Work out the finished part from the listing and answer in its coordinate system (mm). A direction names the side the tool comes from. Coordinates: 2 decimals unless noted, no trailing zeros. Order: outer loops, then holes, each group sorted by start corner. A loop starts at its lowest first (then second) coordinate and runs counter-clockwise, first axis right, second up. Notation, with made-up numbers: M 40.5,-20.75 L 62.5,-20.75 A8 cw 62.5,-14.75 Z; hole C -34.75,5.5 d2. An arc over 180 degrees is marked long. Use a Markdown table: item, result.
from build123d import *

# Parameters (mm, degrees)
F3_DEPTH = 0.5
F4_DEPTH = 0.5
F2_R     = 11.884128
F5_DEPTH = 0.5
F6_R     = 4.759852
F7_DEPTH = 1


with BuildPart() as f3:
    # F0 (on Front) → F3 (new body, symmetric)
    with BuildSketch(Plane.XZ):
        Polygon((0.76961, 25.458554), (-0.685163, 25.458554), (-11.722775, 0), (11.791914, 0), align=None)
    extrude(amount=F3_DEPTH, both=True)

    # F1 (on Right) → F4 (join, symmetric)
    with BuildSketch(Plane.YZ):
        Polygon((0, 25.482798), (-0.616243, 25.482798), (-10.725138, 0), (0, 0), (11.086991, 0), (0.637034, 25.482798), align=None)
    extrude(amount=F4_DEPTH, both=True)

    # F2 (on Top) → F5 (join)
    with BuildSketch(Plane.XY):
        Circle(F2_R)
    extrude(amount=-F5_DEPTH)

    # F6 (on face) → F7 (join)
    with BuildSketch(Plane.XY.offset(25.482798)):
        Circle(F6_R)
    extrude(amount=F7_DEPTH)


solid = f3.part
(1) A cutting plane is placed at D-D (x = 0). Determine the outline of the cut face in (y, z), then the cut area to 3 significant figures.
Conclusion:
| item | result |
|---|---|
| outline | M -11.88,-0.5 L 11.88,-0.5 L 11.88,0 L 11.09,0 L 0.64,25.48 L 4.76,25.48 L 4.76,26.48 L -4.76,26.48 L -4.76,25.48 L -0.62,25.48 L -10.73,0 L -11.88,0 Z |
| area | 315 mm2 |
(2) Straight lines are drawn through the part: L1, parallel to Z at x = -1, y = -2.25; L2, parallel to X at y = -5, z = 14; L3, parallel to Z at x = -2.5, y = 4.5. For each, find the intervals that lie inside material, in ascending order.
Conclusion:
| item | result |
|---|---|
| L1 | -0.5 to 0, 25.48 to 26.48 |
| L2 | -0.5 to 0.5 |
| L3 | -0.5 to 0 |
(3) Determine the mould class of faces 1 (the flat face through (0, 0, 26.483)), 2 (the flat face through (0.007, 5.935, 12.563)), 3 (the flat face through (0, 0, -0.5)), 4 (the cylindrical face through (4.54, 1.43, 25.98)) for opening direction Z: pulls with the +Z half, pulls with the -Z half, needs draft (parallel to the pull), parting line crosses it, or undercut.
Conclusion:
| item | result |
|---|---|
| face 1 | pulls with the +Z half |
| face 2 | undercut |
| face 3 | pulls with the -Z half |
| face 4 | needs draft |
(4) A cutting plane is placed at B-B (x = -3.25). Determine the outline of the cut face in (y, z), then the cut area to 3 significant figures.
Conclusion:
| item | result |
|---|---|
| outline | M -11.43,-0.5 L 11.43,-0.5 L 11.43,0 L 0.5,0 L 0.5,19.54 L -0.5,19.54 L -0.5,0 L -11.43,0 Z; M -3.48,25.48 L 3.48,25.48 L 3.48,26.48 L -3.48,26.48 Z |
| area | 37.9 mm2 |
(5) A cutting plane is placed at A-A (y = 2.25). Determine the outline of the cut face in (x, z).
Conclusion:
| item | result |
|---|---|
| outline | M -11.67,-0.5 L 11.67,-0.5 L 11.67,0 L 0.5,0 L 0.5,21.55 L -0.5,21.55 L -0.5,0 L -11.67,0 Z; M -4.19,25.48 L 4.19,25.48 L 4.19,26.48 L -4.19,26.48 Z |
(6) Given P1, Ø3.5, axis at x = 7.5, z = 8, coming from the -Y side; P2, Ø5, axis at x = -7.5, z = 7.5, coming from the +Y side; P3, Ø8, axis at y = -0.5, z = 17.5, coming from the -X side; P4, Ø7, axis at x = 5.5, y = 0.5, coming from the +Z side, each flat-ended and moving along its own axis, determine where each tip first touches the part or whether it passes through.
Conclusion:
| item | result |
|---|---|
| P1 | y = -0.5 |
| P2 | y = 0.5 |
| P3 | x = -5.87 |
| P4 | z = 26.48 |
(7) Which of the six approach directions +Z, -Z, +X, -X, +Y, -Y give full straight-line access (tool end or side, diameter ignored) to faces 5 (the flat face through (5, -0.5, 10)), 6 (the flat face through (-4, -0.5, 7)), 7 (the flat face through (-4, 0.5, 7))?
Conclusion:
| item | result |
|---|---|
| face 5 | +X, -Y |
| face 6 | -X, -Y |
| face 7 | -X, +Y |
(8) A cutting plane is placed at C-C (z = 4.5). Determine the outline of the cut face in (x, y).
Conclusion:
| item | result |
|---|---|
| outline | M -9.77,-0.5 L -0.5,-0.5 L -0.5,-8.94 L 0.5,-8.94 L 0.5,-0.5 L 9.84,-0.5 L 9.84,0.5 L 0.5,0.5 L 0.5,9.24 L -0.5,9.24 L -0.5,0.5 L -9.77,0.5 Z |
